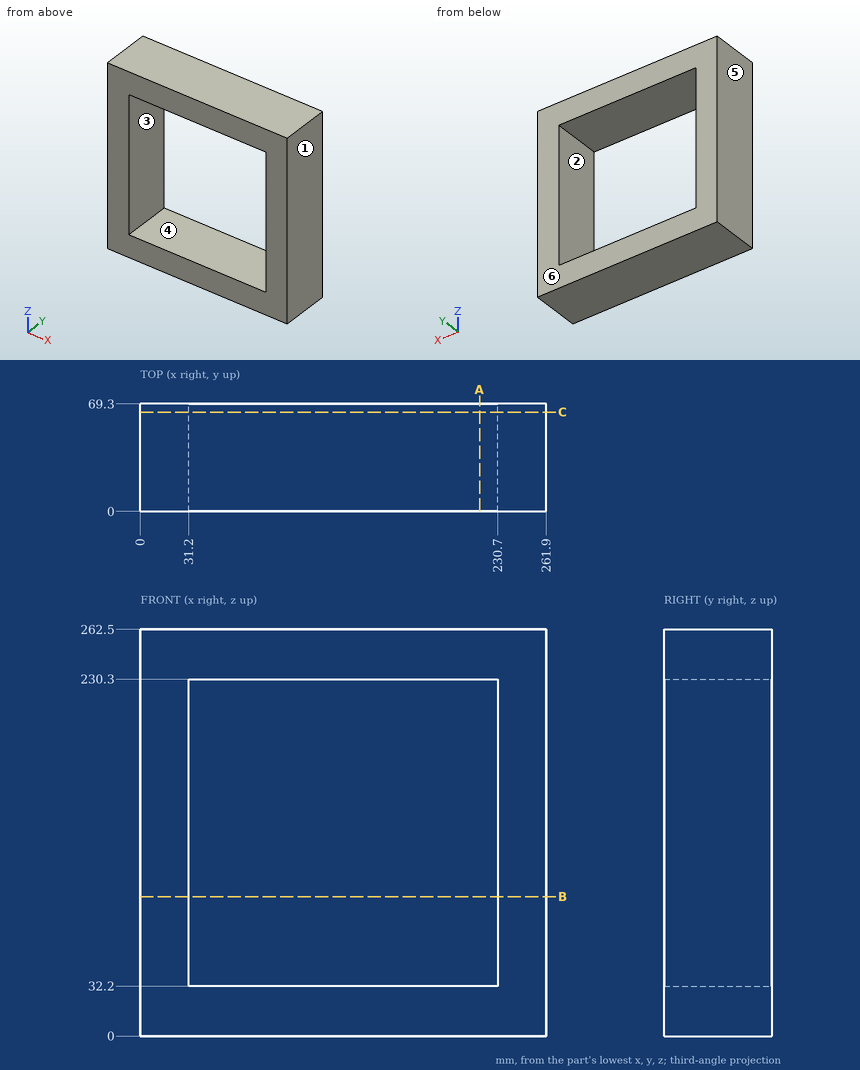
Input: dimensioned drawing with shaded views. Units: mm. Origin: part minimum x, y, z. A direction names the side the tool comes from. Give positions to 0.01 mm unless a question says otherwise; leave off trailing zeros. Order: outer loops, then holes, each group sorted by start corner. A loop starts at its lowest first (then second) coordinate and runs counter-clockwise, first axis right, second up. Notation, with made-up numbers: (42, 89.25) -> (63, 89.25) arc R22 ccw to (63, 119.25) -> close; hole circle Ø8 at (80, 16). An arc over 180 degrees is marked (long way). Use a Markdown table: item, result.
1) Section query A-A, the plane x = 219. Return the cut outline in (y, z), then the cut area to 3 significant figures.
Answer list:
| item | result |
|---|---|
| outline | (0, 0) -> (69.3, 0) -> (69.3, 32.2) -> (0, 32.2) -> close; (0, 230.3) -> (69.3, 230.3) -> (69.3, 262.5) -> (0, 262.5) -> close |
| area | 4,460 mm² |
2) Section query B-B, the plane z = 90. Return the cut outline in (x, y), then the cut area to 3 significant figures.
Answer list:
| item | result |
|---|---|
| outline | (0, 0) -> (31.2, 0) -> (31.2, 69.3) -> (0, 69.3) -> close; (230.7, 0) -> (261.9, 0) -> (261.9, 69.3) -> (230.7, 69.3) -> close |
| area | 4,320 mm² |
3) Mould query, pull axis X, two halves, no side actions, for the marked faces 3, 4, 5 and 6. Classes: +X half, -X half, draft (parallel to the pull), parting line (faces both ways), or undercut.
Answer list:
| item | result |
|---|---|
| face 3 | undercut |
| face 4 | undercut |
| face 5 | -X half |
| face 6 | draft |
4) Reachability of the marked faces 1 and 2 from +Z, -Z, +X, -X, +Y, -Y: full face, straight path, thin tool, end or side. Return the list, or none.
Answer list:
| item | result |
|---|---|
| face 1 | +Z, -Z, +X, +Y, -Y |
| face 2 | +Y, -Y |
5) Ray query, line 1 along Z through (x, y) = (48, 39); line 2 along X through (y, z) = (5, 88). Return the intervals inside material, ascending. Write a range as [from, to].
Answer list:
| item | result |
|---|---|
| line 1 | [0, 32.2], [230.3, 262.5] |
| line 2 | [0, 31.2], [230.7, 261.9] |
6) Section query C-C, the plane y = 64. Return the cut outline in (x, z).
Answer list:
| item | result |
|---|---|
| outline | (0, 0) -> (261.9, 0) -> (261.9, 262.5) -> (0, 262.5) -> close; hole (31.2, 32.2) -> (230.7, 32.2) -> (230.7, 230.3) -> (31.2, 230.3) -> close |
